from build123d import *

# Parameters (mm, degrees)
SKETCH_W      = 107.45
SKETCH_H      = 61.527006
SKETCH_R      = 1.7
PAD_DEPTH     = 2
SKETCH001_R   = 3.3
SKETCH001_R_2 = 1.7
SKETCH001_R_3 = 2.5
PAD001_DEPTH  = 3
SKETCH002_W   = 1.6
SKETCH002_H   = 18.027006
PAD002_DEPTH  = 10


with BuildPart() as part:
    # Sketch → Pad (new body)
    with BuildSketch(Plane.XY):
        Rectangle(SKETCH_W, SKETCH_H)
        with Locations((46.725, -24.063503)):
            Circle(SKETCH_R, mode=Mode.SUBTRACT)
        with Locations((-36.025, -24.063503)):
            Circle(SKETCH_R, mode=Mode.SUBTRACT)
        with Locations((16.29071, -19.66845)):
            Circle(SKETCH_R, mode=Mode.SUBTRACT)
        with Locations((-34.537088, 24.063503)):
            Circle(SKETCH_R, mode=Mode.SUBTRACT)
        with Locations((40.512912, 24.063503)):
            Circle(SKETCH_R, mode=Mode.SUBTRACT)
        with Locations((16.29071, 9.045682)):
            Circle(SKETCH_R, mode=Mode.SUBTRACT)
    extrude(amount=PAD_DEPTH)

    # Sketch001 → Pad001 (join)
    with BuildSketch(Plane.XY.offset(2)):
        with Locations((16.29071, 9.045682)):
            Circle(SKETCH001_R)
        with Locations((16.29071, 9.045682)):
            Circle(SKETCH001_R_2, mode=Mode.SUBTRACT)
        with Locations((40.512912, 24.063503)):
            Circle(SKETCH001_R_3)
        with Locations((40.512912, 24.063503)):
            Circle(SKETCH001_R_2, mode=Mode.SUBTRACT)
        with Locations((46.725, -24.063503)):
            Circle(SKETCH001_R)
        with Locations((46.725, -24.063503)):
            Circle(SKETCH001_R_2, mode=Mode.SUBTRACT)
        with Locations((16.29071, -19.66845)):
            Circle(SKETCH001_R)
        with Locations((16.29071, -19.66845)):
            Circle(SKETCH001_R_2, mode=Mode.SUBTRACT)
        with Locations((-36.025, -24.063503)):
            Circle(SKETCH001_R)
        with Locations((-36.025, -24.063503)):
            Circle(SKETCH001_R_2, mode=Mode.SUBTRACT)
        with Locations((-34.537088, 24.063503)):
            Circle(SKETCH001_R_3)
        with Locations((-34.537088, 24.063503)):
            Circle(SKETCH001_R_2, mode=Mode.SUBTRACT)
    extrude(amount=PAD001_DEPTH)

    # Sketch002 → Pad002 (join)
    with BuildSketch(Plane.XY):
        Polygon((-53.725, 30.763503), (53.725, 30.763503), (53.725, -30.763503), (-53.725, -30.763503), (-53.725, -22.763503), (-55.325, -22.763503), (-55.325, -32.363503), (55.325, -32.363503), (55.325, 32.363503), (-55.325, 32.363503), (-55.325, 23.263503), (-53.725, 23.263503), align=None)
        with Locations((-54.525, -0.75)):
            Rectangle(SKETCH002_W, SKETCH002_H)
    extrude(amount=PAD002_DEPTH)


solid = part.part
Could you check a few things on this model? Use its own coordinates, in mm. A direction names the side the tool comes from. Coordinates: 2 decimals unless noted, no trailing zeros. Write each loop counter-clockwise with the first axis right and the second up, starting at its lowest first coordinate (ties: lowest second). Pieces come first, ordered by that corner, then holes. Notation, with made-up numbers: (-31, -20.75) - (4, -20.75) arc R32 ccw to (4, 9.25) - close; hole circle Ø9 at (24.5, -29). An arc over 180 degrees is marked (long way). Write item = value, one per line.
1) Will these pins go through, and if not, where does the flat tip stop? pin 1 Ø2.5 at (x, y) = (40.5, 25) entering from +Z; pin 2 Ø1.5 at (x, y) = (-8.5, 18.5) entering from +Z; pin 3 Ø1.6 at (y, z) = (-14.5, 1) entering from -X (3 decimals).
Result set:
pin_1 = 5
pin_2 = 2
pin_3 = -53.725
2) Suppose I cut it at B-B on y = 0.5. Please give me the cut outline in (x, z) (3 decimals), plus the area to 3 significant figures.
Result set:
outline = (-55.325, 0) - (55.325, 0) - (55.325, 10) - (53.725, 10) - (53.725, 2) - (-53.725, 2) - (-53.725, 10) - (-55.325, 10) - close
area = 247 mm2
3) Suppose I cut it at C-C on x = -2. Please give me the cut outline in (y, z), plus the area to 3 significant figures.
Result set:
outline = (-32.36, 0) - (32.36, 0) - (32.36, 10) - (30.76, 10) - (30.76, 2) - (-30.76, 2) - (-30.76, 10) - (-32.36, 10) - close
area = 155 mm2
4) For faces 1 (the flat face through (55.325, 0, 5)), 2 (the flat face through (-53.725, 27, 6)), 3 (the flat face through (-53.725, 16, 1)), which set-ups out of +Z, -Z, +X, -X, +Y, -Y let a thin tool reach every point of the face, with its end or its side?
Result set:
face_1 = +Z, -Z, +X, +Y, -Y
face_2 = +Z
face_3 = +Z, -Z, -X
5) Suppose I cut it at A-A on z = 7.5. Please give me the cut outline in (x, y) (1 decimal).
Result set:
outline = (-55.3, -32.4) - (55.3, -32.4) - (55.3, 32.4) - (-55.3, 32.4) - (-55.3, 23.3) - (-53.7, 23.3) - (-53.7, 30.8) - (53.7, 30.8) - (53.7, -30.8) - (-53.7, -30.8) - (-53.7, -22.8) - (-55.3, -22.8) - close; (-55.3, -9.8) - (-53.7, -9.8) - (-53.7, 8.3) - (-55.3, 8.3) - close
6) We'd pull the mould along X, two halves only. Please class faces 4 (the flat face through (0, 31, 10)), 5 (the flat face through (-38, -23, 5)), 6 (the flat face through (-55.325, -1, 5)): +X half, -X half, draft (parallel to the pull), parting line (faces both ways), or undercut.
Result set:
face_4 = draft
face_5 = undercut
face_6 = -X half
7) Please list where these lines run through material, in increasing order: line 1 (Y direction, x = -32, z = 9); line 2 (X direction, y = -7.5, z = 3) (3 decimals); line 3 (X direction, y = -25.5, z = 1.75) (3 decimals). Write a range as [from, to].
Result set:
line_1 = [-32.36, -30.76], [30.76, 32.36]
line_2 = [-55.325, -53.725], [53.725, 55.325]
line_3 = [-55.325, -36.934], [-35.116, 45.816], [47.634, 55.325]
